For this review, take the finished solid that the model builds, in its own axes (mm). Face numbers are marked on the shaded views. Give positions to 0.01 mm unless a question says otherwise; leave off trailing zeros. Write each loop counter-clockwise with the first axis right and the second up, starting at its lowest first coordinate (ties: lowest second). Pieces come first, ordered by that corner, then holes. Notation, with made-up numbers: (13, 2.5) -> (22, 2.5) arc R18 ccw to (22, 17.5) -> close; hole circle Ø9 at (28, -1.75). An arc over 180 degrees is marked (long way). Return JSON: item names as keys, results as strings.
Autodesk Inventor part; units mm, degrees
ref_plane "cp1_XY" through (25.4571, 10.2553, 0) normal (1, 0, 0) x (0, 0, -1)
ref_plane "cp1_YZ" through (25.4571, 10.2553, 0) normal (0, 0, -1) x (0, 1, 0)
ref_plane "cp1_ZX" through (25.4571, 10.2553, 0) normal (0, 1, 0) x (1, 0, 0)
sketch "Sketch_1" plane through (0, 0, 0) normal (0, 0, 1) x (1, 0, 0)
  line L0 (50.9143, 0) -> (0, 0)
  arc A0 (-0.6395, 9.3472) -> (-0.6395, 9.1676) centre (-0.5497, 9.2574) ccw
  line L1 (-0.6395, 9.1676) -> (-0.381, 8.9091)
  line L2 (-0.381, 8.9091) -> (0, 8.9091)
  line L3 (0, 8.9091) -> (0.762, 9.671)
  line L4 (0.762, 9.671) -> (50.1523, 9.671)
  line L5 (50.1523, 9.671) -> (50.9143, 8.9091)
  line L6 (50.9143, 8.9091) -> (51.2953, 8.9091)
  line L7 (51.2953, 8.9091) -> (51.5538, 9.1676)
  arc A1 (51.5538, 9.1676) -> (51.5538, 9.3472) centre (51.464, 9.2574) ccw
  line L8 (51.5538, 9.3472) -> (50.8689, 10.0321)
  arc A2 (50.8689, 10.0321) -> (50.3301, 10.2553) centre (50.3301, 9.4933) ccw
  line L9 (50.3301, 10.2553) -> (0.5842, 10.2553)
  arc A3 (0.5842, 10.2553) -> (0.0454, 10.0321) centre (0.5842, 9.4933) ccw
  line L10 (0.0454, 10.0321) -> (-0.6395, 9.3472)
revolve "Revolution1" add sketch "Sketch_1" angle 360 about axis through (50.9143, 0, 0) along (1, 0, 0)
sketch "Sketch_7" plane through (0, 0, 0) normal (0, 0, 1) x (1, 0, 0)
  circle A0 centre (42.1513, 0) radius 1.1938
extrude "Extrusion1" cut sketch "Sketch_7" along normal blind 10.2553
ref_plane "cp1_XY" through (25.4571, 10.2553, 0) normal (1, 0, 0) x (0, 0, -1)
ref_plane "cp1_YZ" through (25.4571, 10.2553, 0) normal (0, 0, -1) x (0, 1, 0)
ref_plane "cp1_ZX" through (25.4571, 10.2553, 0) normal (0, 1, 0) x (1, 0, 0)
ref_plane "cp2_XY" through (25.4571, 0, -10.2553) normal (1, 0, 0) x (0, 0, -1)
ref_plane "cp2_YZ" through (25.4571, 0, -10.2553) normal (0, 0, -1) x (0, 1, 0)
ref_plane "cp2_ZX" through (25.4571, 0, -10.2553) normal (0, 1, 0) x (1, 0, 0)
ref_plane "cp3_XY" through (25.4571, -10.2553, 0) normal (1, 0, 0) x (0, 0, -1)
ref_plane "cp3_YZ" through (25.4571, -10.2553, 0) normal (0, 0, -1) x (0, 1, 0)
ref_plane "cp3_ZX" through (25.4571, -10.2553, 0) normal (0, 1, 0) x (1, 0, 0)
ref_plane "cp4_XY" through (25.4571, 0, 10.2553) normal (1, 0, 0) x (0, 0, -1)
ref_plane "cp4_YZ" through (25.4571, 0, 10.2553) normal (0, 0, -1) x (0, 1, 0)
ref_plane "cp4_ZX" through (25.4571, 0, 10.2553) normal (0, 1, 0) x (1, 0, 0)
ref_plane "tube_front_XY" through (0, 0, 0) normal (1, 0, 0) x (0, 0, -1)
ref_plane "tube_front_YZ" through (0, 0, 0) normal (0, 0, -1) x (0, 1, 0)
ref_plane "tube_front_ZX" through (0, 0, 0) normal (0, 1, 0) x (1, 0, 0)
ref_plane "tube_rear_XY" through (50.9143, 0, 0) normal (1, 0, 0) x (0, 0, -1)
ref_plane "tube_rear_YZ" through (50.9143, 0, 0) normal (0, 0, -1) x (0, 1, 0)
ref_plane "tube_rear_ZX" through (50.9143, 0, 0) normal (0, 1, 0) x (1, 0, 0)
properties part number "04R-2.00453C"
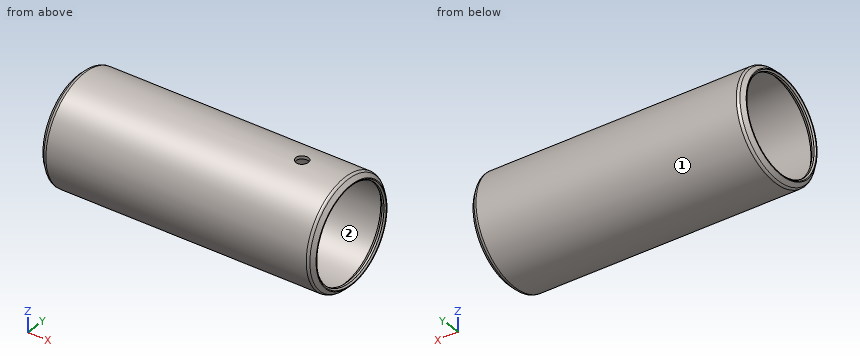
1. For pin 1 (4 mm diameter, centred on x = 23.5, y = -7.5, fed in from -Z); pin 2 (10 mm diameter, centred on x = 6, z = 6, fed in from +Y); pin 3 (1 mm diameter, centred on x = 11.5, y = 6.5, fed in from -Z), all flat-tipped, find the tip position at first contact; note any pin that passes through.
Results found:
{"pin 1": "stops at z = -8.66", "pin 2": "stops at y = 10.21", "pin 3": "stops at z = -8.32"}
2. The part is to be moulded in two halves that separate along Y. For the marked faces 1 and 2, say which applies: +Y half, -Y half, draft (parallel to the pull), parting line (faces both ways), or undercut.
Results found:
{"face 1": "parting line", "face 2": "undercut"}
3. Add section C-C, the plane x = 39.5. State the section outline as (y, z) points, plus the area to 3 significant figures.
Results found:
{"outline": "circle Ø20.51 at (0, 0); hole circle Ø19.34 at (0, 0)", "area": "36.6 mm²"}
4. Add section B-B, the plane y = 0. Count the separate pieces of the cut face and the enclosed holes in it, plus the area to 3 significant figures.
Results found:
{"separate pieces": "3", "enclosed holes": "0", "area": "60.9 mm²"}
5. Add section A-A, the plane z = 0. State the section outline as (x, y) points.
Results found:
{"outline": "(-0.64, -9.35) -> (0.05, -10.03) arc R0.76 ccw to (0.58, -10.26) -> (50.33, -10.26) arc R0.76 ccw to (50.87, -10.03) -> (51.55, -9.35) arc R0.13 ccw to (51.55, -9.17) -> (51.3, -8.91) -> (50.91, -8.91) -> (50.15, -9.67) -> (0.76, -9.67) -> (0, -8.91) -> (-0.38, -8.91) -> (-0.64, -9.17) arc R0.13 ccw to start; (-0.64, 9.17) -> (-0.38, 8.91) -> (0, 8.91) -> (0.76, 9.67) -> (50.15, 9.67) -> (50.91, 8.91) -> (51.3, 8.91) -> (51.55, 9.17) arc R0.13 ccw to (51.55, 9.35) -> (50.87, 10.03) arc R0.76 ccw to (50.33, 10.26) -> (0.58, 10.26) arc R0.76 ccw to (0.05, 10.03) -> (-0.64, 9.35) arc R0.13 ccw to start"}
6. To check wall thickness, follow probe 1 along Z at (x, y) = (24.5, 0); probe 2 along X at (y, z) = (8.75, -4); probe 3 along Z at (x, y) = (24, -7.25). State the ranges of each line that lie inside material, in increasing order.
Results found:
{"probe 1": "z = -10.26 to -9.67, 9.67 to 10.26", "probe 2": "x = -0.37 to 0.71, 50.2 to 51.28", "probe 3": "z = -7.25 to -6.4, 6.4 to 7.25"}
